Input: part model. Units: mm. Frame: model coordinates. Coordinates: 2 decimals unless noted, no trailing zeros. Loops run counter-clockwise (first coordinate to the right, second up) from the corner with the lowest first, then second, coordinate; pieces in that order, holes last. Notation, with made-up numbers: (67, 87.5) - (125, 87.5) arc R18 ccw to (125, 113.5) - close; hole circle Ø11 at (63.25, 44). An arc over 180 degrees is marked (long way). Use a Markdown table: item, result. Add a question column.
1. Section query C-C on y = 50. Return the cut outline in (x, z), then the cut area to 3 significant figures.
2. Section query D-D on x = 52. Return the cut outline in (y, z).
3. Contact query for flat-ended pins moving along their axis: P1, Ø1, axis at y = 69.5, z = -4.5, coming from the +X side; P2, Ø6, axis at x = 52, z = 1.5, coming from the -Y side; P3, Ø2, axis at y = 118, z = -2.5, coming from the +X side. Output: stop coordinate, or through.
4. Section query B-B on z = 3.25. Return the cut outline in (x, y), then the cut area to 3 significant figures.
5. Section query A-A on y = 93. Return the cut outline in (x, z), then the cut area to 3 significant figures.
6. Ray query, L1, parallel to Y at x = 77, z = 3.5; L2, parallel to Y at x = 64, z = -4; L3, parallel to X at y = 84, z = -4. Return the intervals inside material, ascending. Write a range as [from, to].
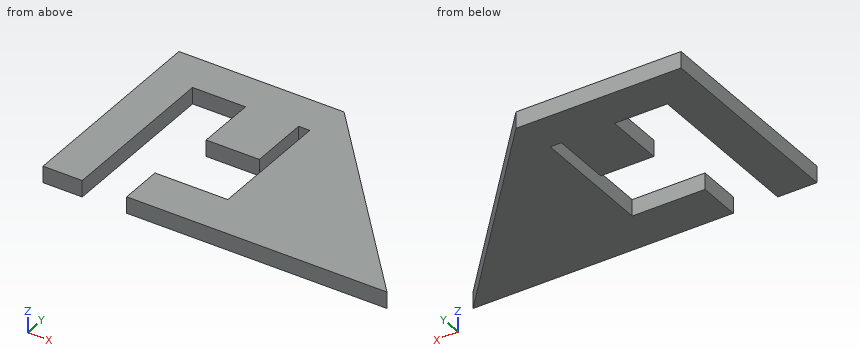
```python
from build123d import *

# Parameters (mm, degrees)
BOSS_EXTRU_1_DEPTH      = 6
BOSS_EXTRU_1_DEPTH_BACK = 6
ENL_V_MAT_EXTRU_1_DEPTH = 292.794448199


with BuildPart() as part:
    # Esquisse1 → Boss.-Extru.1 (new, two sides: drawn at the far end of the back side and taken through both)
    with BuildSketch(Plane.XY.offset(-BOSS_EXTRU_1_DEPTH_BACK)):
        Polygon((0, 0), (250, 0), (120, 150), (0, 150), align=None)
    extrude(amount=BOSS_EXTRU_1_DEPTH + BOSS_EXTRU_1_DEPTH_BACK)

    # Esquisse2 → Enlèv. mat.-Extru.1 (cut, through all)
    with BuildSketch(Plane.XY.offset(6)):
        Polygon((28.515807323, 0), (28.515807323, 121.742691755), (67.012431024, 121.742691755), (67.012431024, 78.36465188), (105.62326997, 78.36465188), (105.62326997, 121.742691755), (113.72405631, 121.742691755), (113.72405631, 31.224508755), (60.816510283, 31.224508755), (60.816510283, 0), align=None)
    extrude(amount=-ENL_V_MAT_EXTRU_1_DEPTH, mode=Mode.SUBTRACT)


solid = part.part
```
Resolved:
| question | item | result |
|---|---|---|
| 1 | outline | (0, -6) - (28.52, -6) - (28.52, 6) - (0, 6) - close; (113.72, -6) - (206.67, -6) - (206.67, 6) - (113.72, 6) - close |
| 1 | area | 1,460 mm² |
| 2 | outline | (121.74, -6) - (150, -6) - (150, 6) - (121.74, 6) - close |
| 3 | P1 | x = 190.2 |
| 3 | P2 | y = 121.74 |
| 3 | P3 | x = 148.6 |
| 4 | outline | (0, 0) - (28.52, 0) - (28.52, 121.74) - (67.01, 121.74) - (67.01, 78.36) - (105.62, 78.36) - (105.62, 121.74) - (113.72, 121.74) - (113.72, 31.22) - (60.82, 31.22) - (60.82, 0) - (250, 0) - (120, 150) - (0, 150) - close |
| 4 | area | 20,700 mm² |
| 5 | outline | (0, -6) - (28.52, -6) - (28.52, 6) - (0, 6) - close; (67.01, -6) - (105.62, -6) - (105.62, 6) - (67.01, 6) - close; (113.72, -6) - (169.4, -6) - (169.4, 6) - (113.72, 6) - close |
| 5 | area | 1,470 mm² |
| 6 | L1 | [0, 31.22], [78.36, 150] |
| 6 | L2 | [0, 31.22], [121.74, 150] |
| 6 | L3 | [0, 28.52], [67.01, 105.62], [113.72, 177.2] |
